Could you check a few things on this model? Use its own coordinates, in mm. A direction names the side the tool comes from. Coordinates: 2 decimals unless noted, no trailing zeros. Write each loop counter-clockwise with the first axis right and the second up, starting at its lowest first coordinate (ties: lowest second). Pieces come first, ordered by that corner, then holes.
Item 1: I want a section at C-C on z = 0. Please give me the cut outline in (x, y), then the cut area to 3 significant figures.
Item 2: If I drill on probe 1 along X at (y, z) = (0.5, 0); probe 2 along Y at (x, z) = (-8.5, -17); probe 3 along X at (y, z) = (-17.75, -10.5), over which ranges is the centre line in solid material (lowest first)?
Item 3: I want a section at A-A on y = -4.75. Please give me the cut outline in (x, z).
Item 4: Thinking about a two-plate mould opening in Z: for faces 4 (the flat face through (0.1, 0.4, -21.463)), 5 (the flat face through (-19.368, -8, -15)), 6 (the flat face through (-20, -7, 8.763)), which applies, +Z half, -Z half, draft (parallel to the pull), parting line (faces both ways), or undercut?
Item 5: I want a section at B-B on x = 0. Please give me the cut outline in (y, z), then the cut area to 3 significant figures.
Item 6: I want a section at D-D on z = -12. Please give me the cut outline in (x, y), then the cut area to 3 significant figures.
Item 7: Which directions (+Z, -Z, +X, -X, +Y, -Y) give clear straight access to the entire face, cutting with the end or side of a thin tool? Please do faces 1 (the flat face through (9, 1.27, 0)), 2 (the flat face through (-19.368, -8, 15)), 3 (the flat face through (-19.368, 1, 0)).
Item 8: For P1, Ø6, axis at x = -9.5, z = 16.5, coming from the -Y side; P2, Ø1.4, axis at y = 0.5, z = -2, coming from the +X side, each with a flat end and sliding along its axis, tell me the tip position at first contact or that it passes through.
from build123d import *

# Parameters (mm, degrees)
SKETCH1_W               = 38.735
SKETCH1_H               = 42.926
BOSS_EXTRUDE1_DEPTH     = 1.27
SKETCH5_R               = 3.96875
SKETCH5_W               = 12.7
SKETCH5_H               = 1.27
BOSS_EXTRUDE3_DEPTH     = 1.27
MIRROR2_COPY_1_SKETCH_R = 3.96875
MIRROR2_COPY_1_SKETCH_W = 12.7
MIRROR2_COPY_1_SKETCH_H = 1.27
MIRROR2_COPY_1_DEPTH    = 1.27
SKETCH6_R               = 7.9375
CUT_EXTRUDE1_DEPTH      = 2.27
CUT_EXTRUDE1_DEPTH_BACK = 22.59


with BuildPart() as part:
    # Sketch1 → Boss-Extrude1 (new body)
    with BuildSketch(Plane(origin=(0, 0, 0), x_dir=(1, 0, 0), z_dir=(0, 1, 0))):
        Rectangle(SKETCH1_W, SKETCH1_H)
    extrude(amount=BOSS_EXTRUDE1_DEPTH)

    # Sketch5 → Boss-Extrude3 (add)
    with BuildSketch(Plane(origin=(19.3675, 0, 0), x_dir=(0, 0, -1), z_dir=(1, 0, 0))):
        with BuildLine():
            Line((-8.763, 0), (-21.463, 0))
            Line((-21.463, 0), (-21.463, -15.24))
            ThreePointArc((-21.463, -15.24), (-15.113, -21.59), (-8.763, -15.24))
            Line((-8.763, -15.24), (-8.763, 0))
        make_face()
        with Locations((-15.113, -15.24)):
            Circle(SKETCH5_R, mode=Mode.SUBTRACT)
        with Locations((-15.113, 0.635)):
            Rectangle(SKETCH5_W, SKETCH5_H)
    boss_extrude3 = extrude(amount=BOSS_EXTRUDE3_DEPTH)

    # Mirror1: Boss-Extrude3 across plane
    add(boss_extrude3.mirror(Plane.XY))

    # Mirror2: Boss-Extrude3 across plane
    add(boss_extrude3.mirror(Plane(origin=(0, 0, 0), x_dir=(0, 0, 1), z_dir=(1, 0, 0))))

    # Mirror2 copy 1 sketch → Mirror2 copy 1 (add)
    with BuildSketch(Plane.ZY.offset(19.3675)):
        with BuildLine():
            Line((-8.763, 0), (-21.463, 0))
            Line((-21.463, 0), (-21.463, -15.24))
            ThreePointArc((-21.463, -15.24), (-15.113, -21.59), (-8.763, -15.24))
            Line((-8.763, -15.24), (-8.763, 0))
        make_face()
        with Locations((-15.113, -15.24)):
            Circle(MIRROR2_COPY_1_SKETCH_R, mode=Mode.SUBTRACT)
        with Locations((-15.113, 0.635)):
            Rectangle(MIRROR2_COPY_1_SKETCH_W, MIRROR2_COPY_1_SKETCH_H)
    extrude(amount=MIRROR2_COPY_1_DEPTH)

    # Sketch6 → Cut-Extrude1 (cut, two sides)
    with BuildSketch(Plane(origin=(0, 0, 0), x_dir=(1, 0, 0), z_dir=(0, 1, 0))) as cut_extrude1_sk:
        Circle(SKETCH6_R)
    extrude(amount=CUT_EXTRUDE1_DEPTH, mode=Mode.SUBTRACT)
    extrude(cut_extrude1_sk.sketch, amount=-CUT_EXTRUDE1_DEPTH_BACK, mode=Mode.SUBTRACT)


solid = part.part
Response values:
1. outline: (-19.37, 0) - (-7.94, 0) - (-7.94, 1.27) - (-19.37, 1.27) - close; (7.94, 0) - (19.37, 0) - (19.37, 1.27) - (7.94, 1.27) - close
1. area: 29.0 mm2
2. probe 1: x = -19.37 to -7.94, 7.94 to 19.37
2. probe 2: y = 0 to 1.27
2. probe 3: x = -20.64 to -19.37, 19.37 to 20.64
3. outline: (-20.64, -21.46) - (-19.37, -21.46) - (-19.37, -8.76) - (-20.64, -8.76) - close; (-20.64, 8.76) - (-19.37, 8.76) - (-19.37, 21.46) - (-20.64, 21.46) - close; (19.37, -21.46) - (20.64, -21.46) - (20.64, -8.76) - (19.37, -8.76) - close; (19.37, 8.76) - (20.64, 8.76) - (20.64, 21.46) - (19.37, 21.46) - close
4. face 4: -Z half
4. face 5: draft
4. face 6: undercut
5. outline: (0, -21.46) - (1.27, -21.46) - (1.27, -7.94) - (0, -7.94) - close; (0, 7.94) - (1.27, 7.94) - (1.27, 21.46) - (0, 21.46) - close
5. area: 34.4 mm2
6. outline: (-20.64, -20.77) - (-19.37, -20.77) - (-19.37, -17.7) - (-20.64, -17.7) - close; (-20.64, -12.78) - (-19.37, -12.78) - (-19.37, 0) - (19.37, 0) - (19.37, -12.78) - (20.64, -12.78) - (20.64, 1.27) - (-20.64, 1.27) - close; (19.37, -20.77) - (20.64, -20.77) - (20.64, -17.7) - (19.37, -17.7) - close
6. area: 92.7 mm2
7. face 1: +Z, -Z, +X, -X, +Y
7. face 2: +Z, -Z, -Y
7. face 3: -X, +Y, -Y
8. P1: stops at y = 0
8. P2: stops at x = 19.37
